For this review, take the finished solid that the model builds, in its own axes (mm). A direction names the side the tool comes from. Coordinates: 2 decimals unless noted, no trailing zeros. Loops run counter-clockwise (first coordinate to the right, second up) from the corner with the lowest first, then second, coordinate; pieces in that order, holes last. Notation, with made-up numbers: (33.25, -24) -> (72.25, -24) arc R9 ccw to (72.25, -8) -> close; hole circle Ø4 at (34.5, -4). An arc over 180 degrees is marked (long way). Answer in a Markdown table with one row per item.
from build123d import *

# Parameters (mm, degrees)
BOSS_EXTRUDE1_DEPTH      = 2.5
BOSS_EXTRUDE1_DEPTH_BACK = 2
SKETCH1_R                = 45
SKETCH2_R                = 45
SKETCH2_R_2              = 42.5
BOSS_EXTRUDE2_DEPTH      = 6
SKETCH3_R                = 4
BOSS_EXTRUDE3_DEPTH      = 16
SKETCH4_R                = 4
SKETCH4_R_2              = 3.5
CUT_EXTRUDE1_DEPTH       = 1.27
CUT_EXTRUDE2_START       = -1.27
SKETCH5_R                = 4
SKETCH5_R_2              = 3.5
CUT_EXTRUDE2_DEPTH       = 1.27
CUT_EXTRUDE3_DEPTH       = 2
SKETCH7_R                = 3.75
CUT_EXTRUDE4_DEPTH       = 66.620118866
SKETCH8_R                = 22.5
SKETCH8_R_2              = 13.5
CUT_EXTRUDE5_DEPTH       = 1
FILLET2_R                = 1.5
SKETCH11_R               = 6.5
BOSS_EXTRUDE4_DEPTH      = 7.127
FILLET3_R                = 2.5


with BuildPart() as part:
    # Sketch1 → Boss-Extrude1 (new, two sides: drawn at the far end of the back side and taken through both)
    with BuildSketch(Plane.XY.offset(-BOSS_EXTRUDE1_DEPTH_BACK)):
        Circle(SKETCH1_R)
    extrude(amount=BOSS_EXTRUDE1_DEPTH + BOSS_EXTRUDE1_DEPTH_BACK)

    # Sketch2 → Boss-Extrude2 (add)
    with BuildSketch(Plane.XY.offset(2.5)):
        Circle(SKETCH2_R)
        Circle(SKETCH2_R_2, mode=Mode.SUBTRACT)
    extrude(amount=BOSS_EXTRUDE2_DEPTH)

    # Sketch3 → Boss-Extrude3 (add)
    with BuildSketch(Plane.XY.offset(2.5)):
        Circle(SKETCH3_R)
    extrude(amount=BOSS_EXTRUDE3_DEPTH)

    # Sketch4 → Cut-Extrude1 (cut)
    with BuildSketch(Plane.XY.offset(13.5)):
        Circle(SKETCH4_R)
        Circle(SKETCH4_R_2, mode=Mode.SUBTRACT)
    extrude(amount=CUT_EXTRUDE1_DEPTH, mode=Mode.SUBTRACT)

    # Sketch5 → Cut-Extrude2 (cut)
    with BuildSketch(Plane.XY.offset(7.135).offset(CUT_EXTRUDE2_START)):
        Circle(SKETCH5_R)
        Circle(SKETCH5_R_2, mode=Mode.SUBTRACT)
    extrude(amount=CUT_EXTRUDE2_DEPTH, mode=Mode.SUBTRACT)

    # Sketch6 → Cut-Extrude3 (cut)
    with BuildSketch(Plane(origin=(0, 0, -2), x_dir=(-1, 0, 0), z_dir=(0, 0, -1))):
        Polygon((-6.639528096, 0), (-3.319764048, -5.75), (3.319764048, -5.75), (6.639528096, 0), (3.319764048, 5.75), (-3.319764048, 5.75), align=None)
    extrude(amount=-CUT_EXTRUDE3_DEPTH, mode=Mode.SUBTRACT)

    # Sketch7 → Cut-Extrude4 (cut, through all)
    with BuildSketch(Plane.XY.offset(2.5)):
        with Locations((-21, 21)):
            Circle(SKETCH7_R)
    extrude(amount=-CUT_EXTRUDE4_DEPTH, mode=Mode.SUBTRACT)

    # Sketch8 → Cut-Extrude5 (cut)
    with BuildSketch(Plane.XY.offset(2.5)):
        Circle(SKETCH8_R)
        Circle(SKETCH8_R_2, mode=Mode.SUBTRACT)
    extrude(amount=-CUT_EXTRUDE5_DEPTH, mode=Mode.SUBTRACT)

    # Fillet2
    # the kernel refuses this fillet: 1.5 mm, written as the material it adds along each edge
    with BuildSketch(Plane(origin=(0, 0, 1.5), x_dir=(1, 0, 0), z_dir=(0, -1, 0))) as fillet2_piece_1:
        with BuildLine():
            CenterArc((21.085786438, 1.5), FILLET2_R, 270, 70.528779366)
            Line((21.085786438, 0), (21.085786438, -0.03))
            Line((21.085786438, -0.03), (22.5, -0.03))
            Line((22.5, -0.03), (22.53, 0))
            ThreePointArc((22.53, 0), (22.53, 0.5), (22.528284271, 0.99))
            Line((22.528284271, 0.99), (22.5, 1))
        make_face()
    revolve(axis=Axis((0, 0, 1.5), (0, 0, 1)))
    with BuildSketch(Plane(origin=(0, 0, 1.5), x_dir=(1, 0, 0), z_dir=(0, -1, 0))) as fillet2_piece_2:
        with BuildLine():
            CenterArc((14.914213562, 1.5), FILLET2_R, 199.471220634, 70.528779366)
            Line((13.5, 1), (13.471715729, 0.99))
            ThreePointArc((13.471715729, 0.99), (13.47, 0.5), (13.47, 0))
            Line((13.47, 0), (13.5, -0.03))
            Line((13.5, -0.03), (14.914213562, -0.03))
            Line((14.914213562, -0.03), (14.914213562, 0))
        make_face()
    revolve(axis=Axis((0, 0, 1.5), (0, 0, 1)))

    # Sketch11 → Boss-Extrude4 (add)
    with BuildSketch(Plane(origin=(0, 0, 0), x_dir=(-1, 0, 0), z_dir=(0, 0, -1))):
        Circle(SKETCH11_R)
    extrude(amount=-BOSS_EXTRUDE4_DEPTH)

    # Fillet3
    fillet3_edges = [part.edges().sort_by_distance(p)[0] for p in [
        (6.5, 0, 2.5),
    ]]
    fillet(fillet3_edges, radius=FILLET3_R)


solid = part.part
Item 1: For faces 1 (the cylindrical face through (-33.727, -25.861, 5.458)), 2 (the cylindrical face through (3.233, -1.341, 14.126)), 3 (the flat face through (5.003, -2.835, -1.014)), list the 3-axis set-ups (+Z, -Z, +X, -X, +Y, -Y) from which the entire face can be reached by the end or side of a thin tool; tool diameter is ignored.
Worked answers:
| item | result |
|---|---|
| face 1 | +Z |
| face 2 | none |
| face 3 | -Z |
Item 2: For L1, parallel to Y at x = 0, z = 5.5; L2, parallel to Z at x = -28, y = 16.5; L3, parallel to Y at x = -30.5, z = 5.75, list the stretches that pass through material, from the lowest coordinate up.
Worked answers:
| item | result |
|---|---|
| L1 | -45 to -42.5, -6.5 to 6.5, 42.5 to 45 |
| L2 | -2 to 2.5 |
| L3 | -33.09 to -29.6, 29.6 to 33.09 |
Item 3: Take a section at B-B, the plane z = 12. State the section outline as (x, y) points, and give its area (3 significant figures).
Worked answers:
| item | result |
|---|---|
| outline | circle Ø8 at (0, 0) |
| area | 50.3 mm² |
Item 4: Take a section at A-A, the plane x = -30.5. State the section outline as (y, z) points.
Worked answers:
| item | result |
|---|---|
| outline | (-33.09, -2) -> (33.09, -2) -> (33.09, 8.5) -> (29.6, 8.5) -> (29.6, 2.5) -> (-29.6, 2.5) -> (-29.6, 8.5) -> (-33.09, 8.5) -> close |
Item 5: Insertion check: pin 1 (12 mm diameter, centred on x = 9, z = 16.5, fed in from +Y); pin 2 (12.5 mm diameter, centred on x = -3, y = 0, fed in from -Z); pin 3 (2 mm diameter, centred on y = 14.5, z = 5, fed in from -X); pin 4 (10 mm diameter, centred on x = 25, z = 15.5, fed in from +Y). Each pin has a flat end and moves straight along its axis. Give the tip position at first contact, or say it passes through.
Worked answers:
| item | result |
|---|---|
| pin 1 | y = 2.65 |
| pin 2 | z = -2 |
| pin 3 | x = -42.93 |
| pin 4 | through |
Item 6: The part is to be moulded in two halves that separate along Y. For faces 4 (the flat face through (0, 0, 18.5)), 5 (the cylindrical face through (-0.867, -3.905, 16.609)), 6 (the cylindrical face through (-19.27, 17.673, 0.281)), say which applies: +Y half, -Y half, draft (parallel to the pull), parting line (faces both ways), or undercut.
Worked answers:
| item | result |
|---|---|
| face 4 | draft |
| face 5 | parting line |
| face 6 | undercut |
Item 7: Take a section at C-C, the plane y = 38. State the section outline as (x, z) points, and give its area (3 significant figures).
Worked answers:
| item | result |
|---|---|
| outline | (-24.1, -2) -> (24.1, -2) -> (24.1, 8.5) -> (19.03, 8.5) -> (19.03, 2.5) -> (-19.03, 2.5) -> (-19.03, 8.5) -> (-24.1, 8.5) -> close |
| area | 278 mm² |
